Autodesk Inventor part; units mm, degrees
ref_plane "YZ Plane" through (0, 0, 0) normal (1, 0, 0) x (0, 1, 0)
ref_plane "XZ Plane" through (0, 0, 0) normal (0, 1, 0) x (-1, 0, 0)
ref_plane "XY Plane" through (0, 0, 0) normal (0, 0, 1) x (1, 0, 0)
sketch "スケッチ1" plane through (0, 0, 0) normal (0, 1, 0) x (-1, 0, 0)
  line L0 (341.5, 441.624) -> (-341.5, 441.624)
  line L1 (-341.5, 441.624) -> (-341.5, -441.624)
  line L2 (-341.5, -441.624) -> (341.5, -441.624)
  line L3 (341.5, -441.624) -> (341.5, 441.624)
  line L4 (0, -618.2736) -> (0, 618.2736)
  line L5 (478.1, 0) -> (-478.1, 0)
  point P0 (0, 0)
  point P1 (0, 441.624)
  point P2 (341.5, 0)
  dimension "d0" = 883.248
  dimension "d1" = 683
extrude "押し出し1" add sketch "スケッチ1" along normal blind 338.552
sketch "スケッチ2" plane through (0, 0, 0) normal (0, -1, 0) x (1, 0, 0)
  line L0 (-341.5, 441.624) -> (341.5, 441.624)
  line L1 (249.8123, 441.624) -> (266.1663, 220.287)
  line L2 (266.1663, 220.287) -> (341.5, -367.5482)
  line L3 (341.5, 441.624) -> (341.5, -441.624)
  line L4 (249.8123, 441.624) -> (341.5, 441.624)
  line L5 (341.5, 441.624) -> (341.5, -367.5482)
  line L6 (0, -782.4861) -> (0, 1603.5489)
  line L7 (-249.8123, 441.624) -> (-266.1663, 220.287)
  line L8 (-266.1663, 220.287) -> (-341.5, -367.5482)
  line L9 (-249.8123, 441.624) -> (-341.5, 441.624)
  line L10 (-341.5, 441.624) -> (-341.5, -367.5482)
  point P0 (0, 0)
  point P1 (0, 1262.6867)
  point P2 (-341.5, 441.624)
extrude "押し出し2" cut sketch "スケッチ2" against normal through all
sketch "スケッチ3" plane through (-249.8123, 0, 441.624) normal (0, 0, 1) x (1, 0, 0)
  line L0 (0, 0) -> (499.6245, 0)
  line L1 (0, 0) -> (-91.6877, 278.2714)
  line L2 (-91.6877, 0) -> (-91.6877, 338.552)
  line L3 (-16.354, 0) -> (-91.6877, 0)
  line L4 (0, 0) -> (-91.6877, 0)
  line L5 (-91.6877, 0) -> (-91.6877, 278.2714)
  line L6 (249.8123, 0) -> (249.8123, -75.9213)
  line L7 (499.6245, 0) -> (0, 0)
  line L8 (499.6245, 0) -> (591.3123, 278.2714)
  line L9 (591.3123, 0) -> (591.3123, 338.552)
  line L10 (515.9785, 0) -> (591.3123, 0)
  line L11 (499.6245, 0) -> (591.3123, 0)
  line L12 (591.3123, 0) -> (591.3123, 278.2714)
extrude "押し出し3" cut sketch "スケッチ3" against normal through all
sketch "スケッチ4" plane through (0, 0, 0) normal (1, 0, 0) x (0, 1, 0)
  line L0 (0, 441.624) -> (338.552, 441.624)
  line L1 (0, 441.624) -> (43.0995, 429.1359)
  line L2 (43.0995, 429.1359) -> (216.735, -84.6593)
  line L3 (216.735, -84.6593) -> (12.1682, -441.624)
  line L4 (0, -441.624) -> (278.2714, -441.624)
  line L5 (12.1682, -441.624) -> (0, -441.624)
  line L6 (0, -441.624) -> (0, 441.624)
  line L7 (0, 441.624) -> (338.552, 441.624)
  line L8 (338.552, 220.287) -> (338.552, -367.5482)
  line L9 (338.552, 441.624) -> (338.552, 220.287)
  line L10 (338.552, 220.287) -> (288.8719, 244.2421)
  line L11 (288.8719, 244.2421) -> (177.502, 390.1926)
  line L12 (177.502, 390.1926) -> (43.0995, 429.1359)
  point P0 (0, 0)
extrude "押し出し5" cut sketch "スケッチ4" along normal through all both and the other way through all contours L0 L9 L10 L11 L12 L1
properties part number "add"
Part model, mm, in its own coordinate system. Coordinates: 2 decimals unless noted, no trailing zeros. Loops run counter-clockwise (first coordinate to the right, second up) from the corner with the lowest first, then second, coordinate; pieces in that order, holes last. Notation, with made-up numbers: (18, 29.25) -> (47, 29.25) arc R24 ccw to (47, 56.25) -> close; hole circle Ø6 at (73.25, 78). An arc over 180 degrees is marked (long way). Use a Markdown table: item, result. Add a question column.
Item 1: Band-saw the part on A-A on x = 232.5. Write the cut outline in (y, z), plus the area to 3 significant figures.
Item 2: Band-saw the part on C-C on z = 277. Write the cut outline in (x, y).
Item 3: Probe probe 1 along X at (y, z) = (253.5, 239); probe 2 along Z at (x, y) = (50, 91); probe 3 along Y at (x, z) = (-169.5, 221.5). List the from-to ranges inside material, lowest first.
Item 4: Band-saw the part on D-D on z = 73. Write the cut outline in (x, y).
Item 5: Flat gauge pins, fed straight in: P1, Ø8, axis at y = 133, z = 135, coming from the +X side; P2, Ø4, axis at y = 135, z = 270.5, coming from the -X side; P3, Ø2, axis at y = 171.5, z = 80, coming from the -X side. Where does each tip first touch, or does it go through?
Item 6: Band-saw the part on B-B on y = 241. Write the cut outline in (x, z).
Geometry says:
| question | item | result |
|---|---|---|
| 1 | outline | (0, -441.62) -> (338.55, -441.62) -> (338.55, 220.29) -> (288.87, 244.24) -> (177.5, 390.19) -> (43.1, 429.14) -> (0, 441.62) -> close |
| 1 | area | 270,000 mm² |
| 2 | outline | (-261.98, 36.92) -> (-249.81, 0) -> (249.81, 0) -> (261.98, 36.92) -> (261.98, 263.88) -> (-261.98, 263.88) -> close |
| 3 | probe 1 | -264.78 to 264.78 |
| 3 | probe 2 | -441.62 to 415.26 |
| 3 | probe 3 | 0 to 336.04 |
| 4 | outline | (-285.04, 106.92) -> (-249.81, 0) -> (249.81, 0) -> (285.04, 106.92) -> (285.04, 338.55) -> (-285.04, 338.55) -> close |
| 5 | P1 | x = 277.61 |
| 5 | P2 | x = -262.6 |
| 5 | P3 | x = -284.27 |
| 6 | outline | (-329.22, -441.62) -> (329.22, -441.62) -> (329.22, -271.72) -> (266.17, 220.29) -> (259.76, 306.98) -> (-259.76, 306.98) -> (-266.17, 220.29) -> (-329.22, -271.72) -> close |
